from build123d import *

# Parameters (mm, degrees)
SKETCH1_W               = 20
SKETCH1_H               = 20
BOSS_EXTRUDE1_DEPTH     = 10
SKETCH2_W               = 12
SKETCH2_H               = 12
CUT_EXTRUDE1_DEPTH      = 19
SKETCH3_W               = 12
SKETCH3_H               = 12
CUT_EXTRUDE2_DEPTH      = 31
SKETCH4_W               = 12
SKETCH4_H               = 12
CUT_EXTRUDE3_DEPTH      = 39
CUT_EXTRUDE5_DEPTH      = 21
CUT_EXTRUDE5_DEPTH_BACK = 6
SKETCH5_W               = 16
SKETCH5_H               = 16
CUT_EXTRUDE8_START      = 4
SKETCH6_W               = 17.478582849
SKETCH6_H               = 18.231479144
CUT_EXTRUDE8_DEPTH      = 43
FILLET3_R               = 9
FILLET4_R               = 9
FILLET5_R               = 9
FILLET6_R               = 9
FILLET7_R               = 9
FILLET8_R               = 9
FILLET9_R               = 5
FILLET10_R              = 5
FILLET11_R              = 5
FILLET12_R              = 5
FILLET13_R              = 5
FILLET14_R              = 5


with BuildPart() as part:
    # Sketch1 → Boss-Extrude1 (new, symmetric)
    with BuildSketch(Plane.XY):
        with Locations((10, 10)):
            Rectangle(SKETCH1_W, SKETCH1_H)
    extrude(amount=BOSS_EXTRUDE1_DEPTH, both=True)

    # Sketch2 → Cut-Extrude1 (cut, symmetric)
    with BuildSketch(Plane.XY):
        with Locations((10, 10)):
            Rectangle(SKETCH2_W, SKETCH2_H)
    extrude(amount=CUT_EXTRUDE1_DEPTH, both=True, mode=Mode.SUBTRACT)

    # Sketch3 → Cut-Extrude2 (cut, symmetric)
    with BuildSketch(Plane(origin=(0, 0, 0), x_dir=(1, 0, 0), z_dir=(0, 1, 0))):
        with Locations((10, 0)):
            Rectangle(SKETCH3_W, SKETCH3_H)
    extrude(amount=CUT_EXTRUDE2_DEPTH, both=True, mode=Mode.SUBTRACT)

    # Sketch4 → Cut-Extrude3 (cut, symmetric)
    with BuildSketch(Plane(origin=(0, 0, 0), x_dir=(0, 0, -1), z_dir=(1, 0, 0))):
        with Locations((0, 10)):
            Rectangle(SKETCH4_W, SKETCH4_H)
    extrude(amount=CUT_EXTRUDE3_DEPTH, both=True, mode=Mode.SUBTRACT)

    # Sketch5 → Cut-Extrude5 (cut, two sides: drawn at the far end of the back side and taken through both)
    with BuildSketch(Plane.XY.offset(-CUT_EXTRUDE5_DEPTH_BACK)):
        with Locations((8, 8)):
            Rectangle(SKETCH5_W, SKETCH5_H)
    extrude(amount=CUT_EXTRUDE5_DEPTH + CUT_EXTRUDE5_DEPTH_BACK, mode=Mode.SUBTRACT)

    # Sketch6 → Cut-Extrude8 (cut)
    with BuildSketch(Plane(origin=(0, 0, 0), x_dir=(1, 0, 0), z_dir=(0, 1, 0)).offset(CUT_EXTRUDE8_START)):
        with Locations((12.739291425, 3.115739572)):
            Rectangle(SKETCH6_W, SKETCH6_H)
    extrude(amount=CUT_EXTRUDE8_DEPTH, mode=Mode.SUBTRACT)

    # Fillet3
    fillet3_edges = [part.edges().sort_by_distance(p)[0] for p in [
        (20, 20, 8),
    ]]
    fillet(fillet3_edges, radius=FILLET3_R)

    # Fillet4
    fillet4_edges = [part.edges().sort_by_distance(p)[0] for p in [
        (0, 0, -8),
    ]]
    fillet(fillet4_edges, radius=FILLET4_R)

    # Fillet5
    fillet5_edges = [part.edges().sort_by_distance(p)[0] for p in [
        (20, 2, -10),
    ]]
    fillet(fillet5_edges, radius=FILLET5_R)

    # Fillet6
    fillet6_edges = [part.edges().sort_by_distance(p)[0] for p in [
        (0, 18, 10),
    ]]
    fillet(fillet6_edges, radius=FILLET6_R)

    # Fillet7
    fillet7_edges = [part.edges().sort_by_distance(p)[0] for p in [
        (2, 20, -10),
    ]]
    fillet(fillet7_edges, radius=FILLET7_R)

    # Fillet8
    fillet8_edges = [part.edges().sort_by_distance(p)[0] for p in [
        (18, 0, 10),
    ]]
    fillet(fillet8_edges, radius=FILLET8_R)

    # Fillet9
    fillet9_edges = [part.edges().sort_by_distance(p)[0] for p in [
        (4, 18, 6),
    ]]
    fillet(fillet9_edges, radius=FILLET9_R)

    # Fillet10
    fillet10_edges = [part.edges().sort_by_distance(p)[0] for p in [
        (16, 2, -6),
    ]]
    fillet(fillet10_edges, radius=FILLET10_R)

    # Fillet11
    fillet11_edges = [part.edges().sort_by_distance(p)[0] for p in [
        (16, 16, 8),
    ]]
    fillet(fillet11_edges, radius=FILLET11_R)

    # Fillet12
    fillet12_edges = [part.edges().sort_by_distance(p)[0] for p in [
        (4, 4, -8),
    ]]
    fillet(fillet12_edges, radius=FILLET12_R)

    # Fillet13
    fillet13_edges = [part.edges().sort_by_distance(p)[0] for p in [
        (18, 4, 6),
    ]]
    fillet(fillet13_edges, radius=FILLET13_R)

    # Fillet14
    fillet14_edges = [part.edges().sort_by_distance(p)[0] for p in [
        (2, 16, -6),
    ]]
    fillet(fillet14_edges, radius=FILLET14_R)


solid = part.part
Verification items for the finished model (mm, model axes). A direction names the side the tool comes from. Round coordinates to 2 decimals unless told otherwise and drop trailing zeros. Loops run counter-clockwise (first coordinate to the right, second up) from the corner with the lowest first, then second, coordinate; pieces in that order, holes last. Notation, with made-up numbers: (-38.75, -8.75) - (-21.75, -8.75) arc R11 ccw to (-21.75, 8.25) - close; hole circle Ø1 at (33, -5). An arc over 180 degrees is marked (long way). Write item = value, one per line.
Q1. Material ranges on L1, parallel to Y at x = 3.25, z = 4.75; L2, parallel to Z at x = 9.25, y = 19.25; L3, parallel to Y at x = 13.5, z = -9, recorded low to high.
Here are the results:
L1 = 16 to 20
L2 = 6 to 10
L3 = 0 to 4
Q2. Depth check by flat-ended pin: pin 1 (5 mm diameter, centred on x = 15, y = 15.5, fed in from -Z); pin 2 (5.5 mm diameter, centred on x = 15, z = -3.5, fed in from +Y); pin 3 (10 mm diameter, centred on y = 3.5, z = 6.5, fed in from -X). Enter the tip coordinate at first touch or a pass-through.
Here are the results:
pin_1 = 6
pin_2 = 4
pin_3 = 16
Q3. Sectioned sample at C-C on y = 17.75. Record the boundary of the cut face in (x, z), plus the area to 3 significant figures.
Here are the results:
outline = (0, -6.95) - (4, -6.95) - (4, 1) arc R5 cw to (9, 6) - (16.95, 6) - (16.95, 10) - (9, 10) arc R9 ccw to (0, 1) - close
area = 108 mm^2
Q4. Tool access check on faces 1 (the flat face through (4, 16, 6)), 2 (the flat face through (4, 16, -6)), 3 (the flat face through (16, 0, -6)). Record the directions out of +Z, -Z, +X, -X, +Y, -Y that give a thin tool (end or side, any length) a straight path to the whole face; none if there is none.
Here are the results:
face_1 = +Z, -X, -Y
face_2 = -Z, +X, +Y
face_3 = +Z, -Z, +X, -X, -Y
Q5. Sectioned sample at D-D on z = -8. Record the boundary of the cut face in (x, y).
Here are the results:
outline = (0, 9) arc R9 ccw to (9, 0) - (16.66, 0) - (16.66, 4) - (9, 4) arc R5 cw to (4, 9) - (4, 16.66) - (0, 16.66) - close
Q6. Sectioned sample at B-B on z = -2. Record the boundary of the cut face in (x, y), plus the area to 3 significant figures.
Here are the results:
outline = (0, 15.9) - (4, 15.9) - (4, 19.94) - (0, 19.94) - close; (15.9, 0) - (19.94, 0) - (19.94, 4) - (15.9, 4) - close
area = 32.4 mm^2
Q7. Sectioned sample at A-A on x = 14. Record the boundary of the cut face in (y, z), plus the area to 3 significant figures.
Here are the results:
outline = (0, -9.49) - (4, -9.49) - (4, -5) - (0, -5) - close; (15, 6) - (19.49, 6) - (19.49, 10) - (15, 10) - close
area = 35.9 mm^2
